Read the model definition and answer for the solid it produces. Units are mm, in the model's axes. Face numbers are marked on the shaded views. A direction names the side the tool comes from. Give positions to 0.01 mm unless a question says otherwise; leave off trailing zeros. Loops run counter-clockwise (first coordinate to the right, second up) from the corner with the lowest first, then second, coordinate; pieces in that order, holes last. Notation, with made-up numbers: (49.25, 45) - (60.25, 45) arc R22 ccw to (60.25, 70) - close; hole circle Ø11 at (38, 4). An arc over 180 degrees is marked (long way). Write item = value, one per line.
```python
from build123d import *

# Parameters (mm, degrees)
F2_R = 5


with BuildPart() as f1:
    # F0 (on Front) → F1 (revolve)
    with BuildSketch(Plane.XZ):
        Polygon((0, 22.5), (0, 0), (240, 0), (240, 55), (195, 55), (195.524231, 42.5), (175, 42.5), (175, 55), (100, 55), (60, 22.5), align=None)
    revolve(axis=Axis((-48.28571, 0, 0), (-1, 0, 0)))

    # F2
    f2_edges = [f1.edges().sort_by_distance(p)[0] for p in [
        (240, 0, -55),
    ]]
    fillet(f2_edges, radius=F2_R)


solid = f1.part
```
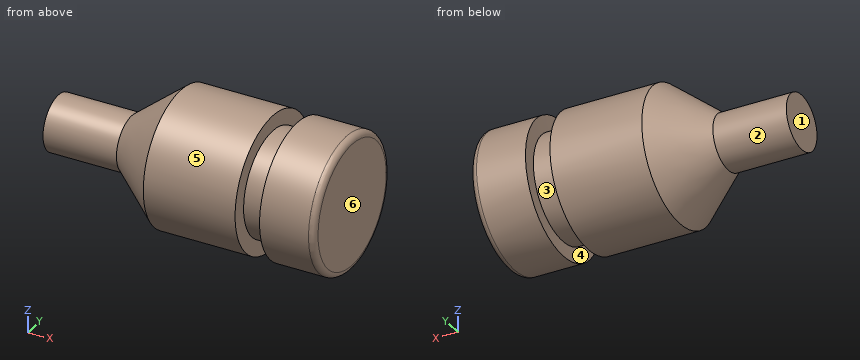
1) A tool of negligible diameter and unlimited length cuts with its end or side. For the marked faces 1, 2 and 3, from which of +Z, -Z, +X, -X, +Y, -Y can it reach the whole face along a straight path? Write none if from no direction.
Output:
face_1 = +Z, -Z, -X, +Y, -Y
face_2 = -X
face_3 = none
2) A cutting plane is placed at D-D on x = 53.5. Determine the outline of the cut face in (y, z), then the cut area to 3 significant figures.
Output:
outline = circle Ø45 at (0, 0)
area = 1,590 mm²
3) Find the intervals of material crossed by probe 1 along Z at (x, y) = (221, -2); probe 2 along X at (y, z) = (45, -21); probe 3 along X at (y, z) = (-29, 39), in increasing order.
Output:
probe_1 = -54.96 to 54.96
probe_2 = 93.43 to 175, 195.22 to 240
probe_3 = 92.12 to 175, 195.27 to 240
4) A cutting plane is placed at C-C on x = 88. Determine the outline of the cut face in (y, z), then the cut area to 3 significant figures.
Output:
outline = circle Ø90.5 at (0, 0)
area = 6,430 mm²
5) The mould has two halves that part along Z. Classify the marked faces 4, 5 and 6: pulls with the +Z half, pulls with the -Z half, needs draft (parallel to the pull), parting line crosses it, or undercut.
Output:
face_4 = undercut
face_5 = parting line crosses it
face_6 = needs draft
6) A cutting plane is placed at A-A on z = 0. Determine the outline of the cut face in (x, y).
Output:
outline = (0, -22.5) - (60, -22.5) - (100, -55) - (175, -55) - (175, -42.5) - (195.52, -42.5) - (195, -55) - (235, -55) arc R5 ccw to (240, -50) - (240, 50) arc R5 ccw to (235, 55) - (195, 55) - (195.52, 42.5) - (175, 42.5) - (175, 55) - (100, 55) - (60, 22.5) - (0, 22.5) - close
7) Each of these flat-tipped pins is pushed along its axis until it touches: P1, Ø4, axis at x = 199, y = -4, coming from the -Z side; P2, Ø4, axis at x = 80, y = 13, coming from the -Z side; P3, Ø8, axis at x = 135.5, z = -1, coming from the +Y side; P4, Ø5, axis at y = -5, z = -14, coming from the -X side. Where does it stop, or does it pass through?
Output:
P1 = -54.96
P2 = -38.35
P3 = 55
P4 = 0
